Here's how the part is built. I have some questions about the finished solid (model axes, mm). A direction names the side the tool comes from. Round coordinates to 2 decimals unless told otherwise and drop trailing zeros. Order: outer loops, then holes, each group sorted by start corner. A loop starts at its lowest first (then second) coordinate and runs counter-clockwise, first axis right, second up. Notation, with made-up numbers: M 35,-33 L 91,-33 A8 ccw 91,-25 Z; hole C 29.25,75.5 d2. An arc over 180 degrees is marked long. Write item = value, one per line. Start each with the question number.
Item 1: I want a section at C-C, the plane x = 45. List the corners of the cut face in (y, z) for me, plus the area to 3 significant figures.
Item 2: We'd pull the mould along Y, two halves only. Please class faces 1 (the face through (6, 50, 1.5)), 2 (the face through (0, 70, 2)): pulls with the +Y half, pulls with the -Y half, needs draft (parallel to the pull), parting line crosses it, or undercut.
Item 3: I want a section at A-A, the plane y = 70. List the corners of the cut face in (x, z) for me.
Item 4: I want a section at B-B, the plane z = 0.5. List the corners of the cut face in (x, y) for me (3 decimals), plus the area to 3 significant figures.
Item 5: Please list where these lines run through material, in increasing order: L1, parallel to Y at x = 0, z = 1.4; L2, parallel to Y at x = 0, z = 0.9; L3, parallel to X at y = 0, z = 1.25.
Item 6: I'm going to push flat-ended pins straight in: P1, Ø1, axis at y = 10.5, z = 1.5, coming from the +X side; P2, Ø1.5, axis at x = -14.5, z = 1.5, coming from the +Y side. Where does each tip first touch, or does it pass through?
Item 7: I want a section at D-D, the plane y = -37. List the corners of the cut face in (x, z) for me, plus the area to 3 significant figures.
Item 8: For faces 3 (the face through (2, 2, -0.8)), 4 (the face through (24.43, 49.24, 1.75)), 5 (the face through (0, 70, 1.2)), which set-ups out of +Z, -Z, +X, -X, +Y, -Y let a thin tool reach every point of the face, with its end or its side?
```python
from build123d import *

# Parameters (mm, degrees)
SKETCH1_R           = 115
SKETCH1_R_2         = 12.6
SKETCH1_R_3         = 1.75
BOSS_EXTRUDE1_DEPTH = 1.2
SKETCH2_R           = 115
SKETCH2_R_2         = 1.75
BOSS_EXTRUDE2_DEPTH = 0.8
SKETCH3_R           = 14.25
SKETCH3_R_2         = 13
CUT_EXTRUDE1_DEPTH  = 0.5
BOSS_EXTRUDE3_START = 0.8
SKETCH4_R           = 115
SKETCH4_R_2         = 1.75
BOSS_EXTRUDE3_DEPTH = 0.8
SKETCH5_R           = 1.25
SKETCH5_W           = 1
SKETCH5_H           = 10
CUT_EXTRUDE2_DEPTH  = 2.8
SKETCH6_W           = 1
SKETCH6_H           = 10
BOSS_EXTRUDE4_DEPTH = 2.3


with BuildPart() as part:
    # Sketch1 → Boss-Extrude1 (new body)
    with BuildSketch(Plane.XY):
        Circle(SKETCH1_R)
        with Locations((0, 70)):
            Circle(SKETCH1_R_2, mode=Mode.SUBTRACT)
        Circle(SKETCH1_R_3, mode=Mode.SUBTRACT)
    extrude(amount=BOSS_EXTRUDE1_DEPTH)

    # Sketch2 → Boss-Extrude2 (add)
    with BuildSketch(Plane.XY.offset(1.2)):
        Circle(SKETCH2_R)
        Circle(SKETCH2_R_2, mode=Mode.SUBTRACT)
    extrude(amount=BOSS_EXTRUDE2_DEPTH)

    # Sketch3 → Cut-Extrude1 (cut)
    # profile 1 of 10: a face of its own
    with BuildSketch(Plane.XY.offset(2)):
        with BuildLine():
            Line((-14.304598289, 45.736382), (-13.304598289, 47.468432807))
            ThreePointArc((-13.304598289, 47.468432807), (-14.429598289, 49.416989966), (-13.304598289, 51.365547124))
            Line((-13.304598289, 51.365547124), (-14.304598289, 53.097597932))
            ThreePointArc((-14.304598289, 53.097597932), (-16.429598289, 49.416989966), (-14.304598289, 45.736382))
        make_face()
    # profile 2 of 10: a face of its own
    with BuildSketch(Plane.XY.offset(2)):
        Polygon((-12.179598289, 49.416989966), (-12.209391902, 49.365385915), (-12.209391902, 45), (-10.43132512, 45), (-10.43132512, 50.98245386), (-6.7751753, 45), (-4.860049204, 45), (-4.860049204, 54.245947266), (-6.638115986, 54.245947266), (-6.638115986, 48.167181455), (-10.351682546, 54.245947266), (-12.209391902, 54.245947266), (-12.209391902, 49.468594016), align=None)
    # profile 3 of 10: a face of its own
    with BuildSketch(Plane.XY.offset(2)):
        with BuildLine():
            Line((-16.304598289, 42.272280384), (-15.304598289, 44.004331192))
            ThreePointArc((-15.304598289, 44.004331192), (-18.429598289, 49.416989966), (-15.304598289, 54.829648739))
            Line((-15.304598289, 54.829648739), (-16.304598289, 56.561699547))
            ThreePointArc((-16.304598289, 56.561699547), (-20.429598289, 49.416989966), (-16.304598289, 42.272280384))
        make_face()
    # profile 4 of 10: a face of its own
    with BuildSketch(Plane.XY.offset(2)):
        with BuildLine():
            Line((-18.304598289, 38.808178769), (-17.304598289, 40.540229577))
            ThreePointArc((-17.304598289, 40.540229577), (-22.429598289, 49.416989966), (-17.304598289, 58.293750354))
            Line((-17.304598289, 58.293750354), (-18.304598289, 60.025801162))
            ThreePointArc((-18.304598289, 60.025801162), (-24.429598289, 49.416989966), (-18.304598289, 38.808178769))
        make_face()
    # profile 5 of 10: a face of its own
    with BuildSketch(Plane.XY.offset(2)):
        with BuildLine():
            ThreePointArc((13.304598289, 51.365547124), (14.429598289, 49.416989966), (13.304598289, 47.468432807))
            Line((13.304598289, 47.468432807), (14.304598289, 45.736382))
            ThreePointArc((14.304598289, 45.736382), (16.429598289, 49.416989966), (14.304598289, 53.097597932))
            Line((14.304598289, 53.097597932), (13.304598289, 51.365547124))
        make_face()
    # profile 6 of 10: a face of its own
    with BuildSketch(Plane.XY.offset(2)):
        with BuildLine():
            ThreePointArc((15.304598289, 54.829648739), (18.429598289, 49.416989966), (15.304598289, 44.004331192))
            Line((15.304598289, 44.004331192), (16.304598289, 42.272280384))
            ThreePointArc((16.304598289, 42.272280384), (20.429598289, 49.416989966), (16.304598289, 56.561699547))
            Line((16.304598289, 56.561699547), (15.304598289, 54.829648739))
        make_face()
    # profile 7 of 10: a face of its own
    with BuildSketch(Plane.XY.offset(2)):
        with BuildLine():
            ThreePointArc((17.304598289, 58.293750354), (22.429598289, 49.416989966), (17.304598289, 40.540229577))
            Line((17.304598289, 40.540229577), (18.304598289, 38.808178769))
            ThreePointArc((18.304598289, 38.808178769), (24.429598289, 49.416989966), (18.304598289, 60.025801162))
            Line((18.304598289, 60.025801162), (17.304598289, 58.293750354))
        make_face()
    # profile 8 of 10: a face of its own
    with BuildSketch(Plane.XY.offset(2)):
        Polygon((-2.963444636, 54.245947266), (-2.963444636, 45), (-1.185377855, 45), (-1.185377855, 48.91174692), (2.726369066, 48.91174692), (2.726369066, 50.452738131), (-1.185377855, 50.452738131), (-1.185377855, 52.704956055), (3.319057993, 52.704956055), (3.319057993, 54.245947266), align=None)
    # profile 9 of 10: a face of its own
    with BuildSketch(Plane.XY.offset(2)):
        with BuildLine():
            Line((12.565005258, 47.844906851), (10.786938477, 48.437595778))
            add(Edge.make_bspline(
                [(8.649554033, 46.540991211), (8.774457906, 46.542804078), (8.960902987, 46.552124821), (9.200761468, 46.603342992), (9.371697205, 46.653314203), (9.536735909, 46.716051803), (9.693353441, 46.796521205), (9.844632955, 46.889011376), (9.987435142, 46.997402051), (10.123671935, 47.119091548), (10.24792915, 47.259733892), (10.363183369, 47.415951417), (10.467995906, 47.588781763), (10.565774579, 47.776770817), (10.680063587, 48.058750047), (10.75051939, 48.282015418), (10.786938477, 48.437595778)],
                knots=[0, 0, 0, 0, 0.12046088, 0.178740623, 0.235724111, 0.291792154, 0.348405626, 0.404978529, 0.462271107, 0.520759571, 0.580529381, 0.642578218, 0.707405436, 0.774920301, 0.846330275, 1, 1, 1, 1], degree=3))
            add(Edge.make_bspline(
                [(6.282502629, 49.737807112), (6.285322977, 49.470306981), (6.297610529, 49.082539498), (6.369602887, 48.589695915), (6.440666935, 48.264864831), (6.532669328, 47.970595781), (6.645226739, 47.70740396), (6.779038197, 47.474979778), (6.933893175, 47.273478116), (7.10587723, 47.100389393), (7.290332212, 46.951570368), (7.486169728, 46.82433845), (7.694568912, 46.719631559), (7.916319835, 46.640528882), (8.233117363, 46.562073655), (8.481308806, 46.539908407), (8.649554033, 46.540991211)],
                knots=[0, 0, 0, 0, 0.177656206, 0.256732639, 0.330177257, 0.398062973, 0.460994883, 0.519731382, 0.575527448, 0.629114465, 0.681254032, 0.732497652, 0.783792002, 0.835623311, 0.888378762, 1, 1, 1, 1], degree=3))
            add(Edge.make_bspline(
                [(8.66066695, 52.82349384), (8.491465901, 52.826075047), (8.242559674, 52.799846285), (7.922640611, 52.727085572), (7.699736188, 52.646106315), (7.49074803, 52.54236084), (7.293294797, 52.416290582), (7.108461861, 52.268387934), (6.93618627, 52.096913588), (6.781592493, 51.898763678), (6.645681991, 51.673529995), (6.532934048, 51.418655469), (6.441392441, 51.136639915), (6.369372519, 50.826818405), (6.298040133, 50.35919413), (6.285308784, 49.991144174), (6.282502629, 49.737807112)],
                knots=[0, 0, 0, 0, 0.114442147, 0.169048205, 0.221995274, 0.274768432, 0.326888881, 0.380476958, 0.434920839, 0.491256742, 0.550390474, 0.612762372, 0.679720015, 0.751074463, 0.828128845, 1, 1, 1, 1], degree=3))
            add(Edge.make_bspline(
                [(10.668400691, 51.282502629), (10.641238914, 51.398054972), (10.587850378, 51.565642196), (10.494156792, 51.777398501), (10.408574753, 51.921779276), (10.317598271, 52.060296222), (10.209906332, 52.186819303), (10.09235562, 52.304658865), (9.964105005, 52.412593655), (9.82668186, 52.508441667), (9.682732574, 52.594604872), (9.529640338, 52.664934387), (9.369443041, 52.721855687), (9.202773529, 52.769483738), (8.965989688, 52.809862605), (8.784209014, 52.826424315), (8.66066695, 52.82349384)],
                knots=[0, 0, 0, 0, 0.129415079, 0.191523435, 0.252186483, 0.312349991, 0.372123769, 0.433096486, 0.493819352, 0.554747395, 0.615749876, 0.676633212, 0.738216912, 0.801141922, 0.865493176, 1, 1, 1, 1], degree=3))
            Line((10.668400691, 51.282502629), (12.446467473, 51.638115986))
            add(Edge.make_bspline(
                [(11.51113026, 53.353209569), (11.618919371, 53.252134624), (11.765446177, 53.081421549), (11.939181695, 52.831726814), (12.062269606, 52.625570238), (12.171970389, 52.4010392), (12.311226739, 52.074446139), (12.396954988, 51.816309851), (12.446467473, 51.638115986)],
                knots=[0, 0, 0, 0, 0.223922581, 0.340367194, 0.461366928, 0.58791332, 0.71930972, 1, 1, 1, 1], degree=3))
            add(Edge.make_bspline(
                [(8.784761194, 54.364485051), (9.05213035, 54.36170592), (9.447480124, 54.337725331), (9.952714034, 54.227961891), (10.305824473, 54.11948993), (10.638318496, 53.976085526), (11.056637945, 53.742604246), (11.338718425, 53.518758054), (11.51113026, 53.353209569)],
                knots=[0, 0, 0, 0, 0.269221899, 0.396222126, 0.519140292, 0.640111566, 0.759624432, 1, 1, 1, 1], degree=3))
            add(Edge.make_bspline(
                [(4.504435847, 49.602599951), (4.503806189, 49.95935967), (4.53809244, 50.480966902), (4.660090028, 51.150009144), (4.790227099, 51.606032572), (4.954122369, 52.032375199), (5.160126736, 52.424803313), (5.398535284, 52.788549361), (5.675745533, 53.116946458), (5.983655723, 53.408518035), (6.31361956, 53.666348484), (6.66871472, 53.882641187), (7.047001045, 54.059546034), (7.448974215, 54.196322464), (8.026435231, 54.330802367), (8.478762466, 54.361874395), (8.784761194, 54.364485051)],
                knots=[0, 0, 0, 0, 0.147853475, 0.216062561, 0.281513739, 0.344147287, 0.405039848, 0.464871931, 0.524079073, 0.582724997, 0.640361728, 0.697328761, 0.754684166, 0.813113061, 0.873014604, 1, 1, 1, 1], degree=3))
            add(Edge.make_bspline(
                [(8.721787996, 45), (8.426367251, 44.997988178), (7.990266773, 45.035933953), (7.432039385, 45.166823587), (7.03995053, 45.29954369), (6.670218657, 45.47557439), (6.319473407, 45.687433116), (5.990266678, 45.939486093), (5.683753354, 46.22746781), (5.405279268, 46.5491846), (5.164468655, 46.902896762), (4.958714021, 47.283621418), (4.792375452, 47.693174913), (4.662454179, 48.131132452), (4.537348729, 48.767470915), (4.504184947, 49.264405834), (4.504435847, 49.602599951)],
                knots=[0, 0, 0, 0, 0.126018891, 0.185824822, 0.244304364, 0.302279211, 0.360195978, 0.418835489, 0.47884239, 0.539358251, 0.600002403, 0.661054814, 0.723669356, 0.788261327, 0.855679185, 1, 1, 1, 1], degree=3))
            add(Edge.make_bspline(
                [(12.565005258, 47.844906851), (12.497380357, 47.615920501), (12.382150303, 47.28238474), (12.179541249, 46.869560595), (12.017716763, 46.586721298), (11.832453107, 46.331624647), (11.634211253, 46.095805011), (11.41707355, 45.884234212), (11.182117383, 45.696459001), (10.931602763, 45.530405863), (10.662620144, 45.390024222), (10.379183478, 45.269124387), (10.078419057, 45.171142401), (9.76232112, 45.0927817), (9.309084503, 45.021757353), (8.959586718, 44.99891792), (8.721787996, 45)],
                knots=[0, 0, 0, 0, 0.137894803, 0.202902916, 0.265167572, 0.325674736, 0.3845661, 0.442763708, 0.500294498, 0.557901352, 0.615910004, 0.675133413, 0.735519841, 0.79825159, 0.862854286, 1, 1, 1, 1], degree=3))
        make_face()
    # profile 10 of 10: a face of its own
    with BuildSketch(Plane.XY.offset(2)):
        with Locations((0, 70)):
            Circle(SKETCH3_R)
        with Locations((0, 70)):
            Circle(SKETCH3_R_2, mode=Mode.SUBTRACT)
    extrude(amount=-CUT_EXTRUDE1_DEPTH, mode=Mode.SUBTRACT)

    # Sketch4 → Boss-Extrude3 (add)
    with BuildSketch(Plane(origin=(0, 0, 0), x_dir=(-1, 0, 0), z_dir=(0, 0, -1)).offset(BOSS_EXTRUDE3_START)):
        Circle(SKETCH4_R)
        Circle(SKETCH4_R_2, mode=Mode.SUBTRACT)
    extrude(amount=-BOSS_EXTRUDE3_DEPTH)

    # Sketch5 → Cut-Extrude2 (cut)
    with BuildSketch(Plane.XY.offset(2)):
        with Locations((0, -21.25)):
            Circle(SKETCH5_R)
        with Locations((-18.40303983, 10.625)):
            Circle(SKETCH5_R)
        with Locations((18.40303983, 10.625)):
            Circle(SKETCH5_R)
        with Locations((0, 18.75)):
            Rectangle(SKETCH5_W, SKETCH5_H)
    extrude(amount=-CUT_EXTRUDE2_DEPTH, mode=Mode.SUBTRACT)

    # Sketch6 → Boss-Extrude4 (add)
    with BuildSketch(Plane(origin=(0, 0, -0.8), x_dir=(-1, 0, 0), z_dir=(0, 0, -1))):
        with Locations((0, 18.75)):
            Rectangle(SKETCH6_W, SKETCH6_H)
    extrude(amount=-BOSS_EXTRUDE4_DEPTH)


solid = part.part
```
Filled in:
q1.outline = M -105.83,-0.8 L 105.83,-0.8 L 105.83,2 L -105.83,2 Z
q1.area = 593 mm^2
q2.face_1 = undercut
q2.face_2 = needs draft
q3.outline = M -91.24,-0.8 L 91.24,-0.8 L 91.24,2 L 14.25,2 L 14.25,1.5 L 13,1.5 L 13,2 L -13,2 L -13,1.5 L -14.25,1.5 L -14.25,2 L -91.24,2 Z; hole M -12.6,0 L 12.6,0 L 12.6,1.2 L -12.6,1.2 Z
q4.outline = C 0,0 d230; hole C -18.403,10.625 d2.5; hole C 0,70 d25.2; hole C 0,0 d3.5; hole C 0,-21.25 d2.5; hole C 18.403,10.625 d2.5
q4.area = 41,000 mm^2
q5.L1 = -115 to -22.5, -20 to -1.75, 1.75 to 115
q5.L2 = -115 to -22.5, -20 to -1.75, 1.75 to 57.4, 82.6 to 115
q5.L3 = -115 to -1.75, 1.75 to 115
q6.P1 = 114.56
q6.P2 = 114.18
q7.outline = M -108.89,-0.8 L 108.89,-0.8 L 108.89,2 L -108.89,2 Z
q7.area = 610 mm^2
q8.face_3 = -Z, +X, -X, +Y, -Y
q8.face_4 = +Z
q8.face_5 = none
